Could you check a few things on this model? Use its own coordinates, in mm. Face numbers are marked on the shaded views. Give positions to 0.01 mm unless a question says otherwise; leave off trailing zeros. Loops run counter-clockwise (first coordinate to the right, second up) from the corner with the lowest first, then second, coordinate; pieces in that order, holes last. Notation, with made-up numbers: (-17.5, 78.5) - (30.5, 78.5) arc R17 ccw to (30.5, 91.5) - close; hole circle Ø10 at (60.5, -31). An arc over 180 degrees is marked (long way). Use CSV: the item, a comma, the result in double quotes.
from build123d import *

# Parameters (mm, degrees)
SKETCH1_R           = 1.55
BOSS_EXTRUDE1_DEPTH = 2
BOSS_EXTRUDE2_DEPTH = 5
BOSS_EXTRUDE2_DRAFT = 20


with BuildPart() as part:
    # Sketch1 → Boss-Extrude1 (new body)
    with BuildSketch(Plane(origin=(0, 0, 0), x_dir=(1, 0, 0), z_dir=(0, 1, 0))):
        with BuildLine():
            Line((14, 24.248711306), (19, 32.908965344))
            ThreePointArc((19, 32.908965344), (17.860130505, 33.541254275), (16.699245775, 34.134076676))
            Line((16.699245775, 34.134076676), (17.790465664, 36.898500396))
            ThreePointArc((17.790465664, 36.898500396), (16.101499604, 40.790465664), (12.209534336, 39.101499604))
            Line((12.209534336, 39.101499604), (11.118314447, 36.337075885))
            ThreePointArc((11.118314447, 36.337075885), (0, 38), (-11.118314447, 36.337075885))
            Line((-11.118314447, 36.337075885), (-12.209534336, 39.101499604))
            ThreePointArc((-12.209534336, 39.101499604), (-16.101499604, 40.790465664), (-17.790465664, 36.898500396))
            Line((-17.790465664, 36.898500396), (-16.699245775, 34.134076676))
            ThreePointArc((-16.699245775, 34.134076676), (-17.860130505, 33.541254275), (-19, 32.908965344))
            Line((-19, 32.908965344), (-14, 24.248711306))
            ThreePointArc((-14, 24.248711306), (0, 28), (14, 24.248711306))
        make_face()
        with Locations(Location((-15, 38, 0), (0, 0, 270))):
            Circle(SKETCH1_R, mode=Mode.SUBTRACT)
        with Locations(Location((15, 38, 0), (0, 0, 270))):
            Circle(SKETCH1_R, mode=Mode.SUBTRACT)
    extrude(amount=BOSS_EXTRUDE1_DEPTH)


with BuildPart() as boss_extrude2_tool:
    # Sketch2 → Boss-Extrude2 (with draft: the straight prism first)
    with BuildSketch(Plane(origin=(0, 2, 0), x_dir=(1, 0, 0), z_dir=(0, 1, 0))):
        with BuildLine():
            ThreePointArc((-12.25592959, 26.282925824), (0, 29), (12.25592959, 26.282925824))
            Line((12.25592959, 26.282925824), (15.636875684, 33.53338812))
            ThreePointArc((15.636875684, 33.53338812), (0, 37), (-15.636875684, 33.53338812))
            Line((-15.636875684, 33.53338812), (-12.25592959, 26.282925824))
        make_face()
    extrude(amount=BOSS_EXTRUDE2_DEPTH)
    # Boss-Extrude2: the draft: its side faces are tilted about the plane it starts from
    boss_extrude2_sides = [boss_extrude2_tool.faces().sort_by_distance(p)[0] for p in [
        (0, 4.5, -29),
        (13.946402637, 4.5, -29.908156972),
        (0, 4.5, -37),
        (-13.946402637, 4.5, -29.908156972),
    ]]
    draft(boss_extrude2_sides, Plane(origin=(0, 2, 0), x_dir=(1, 0, 0), z_dir=(0, 1, 0)), BOSS_EXTRUDE2_DRAFT)


with BuildPart() as part_1:
    add(part.part)

    # Boss-Extrude2: add boss_extrude2_tool
    add(boss_extrude2_tool.part)


solid = part_1.part
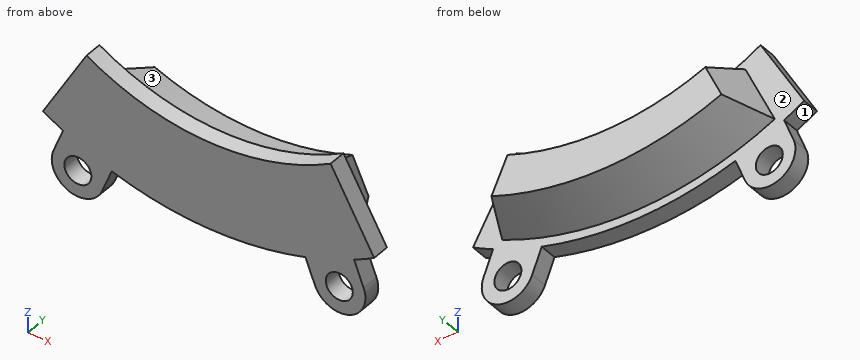
1) Suppose I cut it at A-A (y = 1.25). Please give me the cut outline in (x, z), plus the area to 3 significant figures.
Answer below:
outline,"(-19, -32.91) arc R38 ccw to (-16.7, -34.13) - (-17.79, -36.9) arc R3 ccw to (-12.21, -39.1) - (-11.12, -36.34) arc R38 ccw to (11.12, -36.34) - (12.21, -39.1) arc R3 ccw to (17.79, -36.9) - (16.7, -34.13) arc R38 ccw to (19, -32.91) - (14, -24.25) arc R28 cw to (-14, -24.25) - close; hole circle Ø3.1 at (-15, -38); hole circle Ø3.1 at (15, -38)"
area,"393 mm2"
2) We'd pull the mould along Z, two halves only. Please class the marked faces 1, 2 and 3: +Z half, -Z half, draft (parallel to the pull), parting line (faces both ways), or undercut.
Answer below:
face 1,"undercut"
face 2,"draft"
face 3,"+Z half"
3) Suppose I cut it at B-B (z = -25.25). Please give me the cut outline in (x, y).
Answer below:
outline,"(-14.58, 0) - (-12.1, 0) - (-12.1, 2) - (-14.58, 2) - close; (12.1, 0) - (14.58, 0) - (14.58, 2) - (12.1, 2) - close"
4) I'm going to push flat-ended pins straight in: P1, Ø1.9, axis at x = 15, z = -38, coming from the +Y side; P2, Ø1, axis at x = 6.5, y = 1.5, coming from the -Z side. Where does each tip first touch, or does it pass through?
Answer below:
P1,"passes through"
P2,"stops at z = -37.52"
5) I need wall thicknesses on line 1 along Y through (x, z) = (-14.5, -40); line 2 along Z through (x, y) = (-10, 2.5); line 3 along Z through (x, y) = (-13.5, 2.5). Which ranges of each line are inside material? Lowest first, please.
Answer below:
line 1,"y = 0 to 2"
line 2,"z = -35.43 to -27.42"
line 3,"z = -34.25 to -29.38"
6) Suppose I cut it at D-D (z = -31.25). Please give me the cut outline in (x, y).
Answer below:
outline,"(-18.04, 0) - (18.04, 0) - (18.04, 2) - (14.57, 2) - (12.56, 7) - (-12.56, 7) - (-14.57, 2) - (-18.04, 2) - close"
7) Suppose I cut it at C-C (z = -37.5). Please give me the cut outline in (x, y).
Answer below:
outline,"(-17.96, 0) - (-16.47, 0) - (-16.47, 2) - (-17.96, 2) - close; (-13.53, 0) - (-11.58, 0) - (-11.58, 2) - (-13.53, 2) - close; (-6.14, 0) - (6.14, 0) - (6.14, 2) - (-6.14, 2) - close; (11.58, 0) - (13.53, 0) - (13.53, 2) - (11.58, 2) - close; (16.47, 0) - (17.96, 0) - (17.96, 2) - (16.47, 2) - close"
